Could you check a few things on this model? Use its own coordinates, in mm. A direction names the side the tool comes from. Give positions to 0.01 mm unless a question says otherwise; leave off trailing zeros. Order: outer loops, then holes, each group sorted by start corner. A loop starts at its lowest first (then second) coordinate and runs counter-clockwise, first axis right, second up.
Autodesk Fusion 360 part; units mm, degrees
sketch "Sketch1" plane through (0, 0, 0) normal (0, 0, 1) x (1, 0, 0)
  circle A0 centre (0, 0) radius 5
  circle A1 centre (0, 0) radius 3.575
  dimension "d1" = 10
  dimension "d2" = 7.15
extrude "Extrude1" add sketch "Sketch1" along normal blind 2
extrude "Extrude2" add sketch "Sketch1" along normal blind 4.9 contours A1
hole "Hole1" at (0, 0, 0) direction (0, 0, 1) diameter 5.5 depth 10 tip angle 118
Item 1: We'd pull the mould along X, two halves only. Please class faces 3 (the cylindrical face through (-1.08, 4.88, 0.99)), 4 (the flat face through (3.3, -2.2, 2)), 5 (the cylindrical face through (2.685, -0.596, 2.484)): +X half, -X half, draft (parallel to the pull), parting line (faces both ways), or undercut.
Findings:
face 3: parting line
face 4: draft
face 5: undercut
Item 2: Imagine slicing it at A-A on y = 0. List the corners of the cut face in (x, z) for me (3 decimals), then the cut area to 3 significant figures.
Findings:
outline: (-5, 0) - (-2.75, 0) - (-2.75, 4.9) - (-3.575, 4.9) - (-3.575, 2) - (-5, 2) - close; (2.75, 0) - (5, 0) - (5, 2) - (3.575, 2) - (3.575, 4.9) - (2.75, 4.9) - close
area: 13.8 mm2
Item 3: Imagine slicing it at D-D on y = -3.25. List the corners of the cut face in (x, z) for me.
Findings:
outline: (-3.8, 0) - (3.8, 0) - (3.8, 2) - (1.49, 2) - (1.49, 4.9) - (-1.49, 4.9) - (-1.49, 2) - (-3.8, 2) - close
Item 4: For faces 1 (the cylindrical face through (-0.465, -3.545, 3.43)), 2 (the flat face through (2.2, -2.2, 0)), which set-ups out of +Z, -Z, +X, -X, +Y, -Y let a thin tool reach every point of the face, with its end or its side?
Findings:
face 1: +Z
face 2: -Z, +X, -X, +Y, -Y
Item 5: Please list where these lines run through material, in increasing order: line 1 along Y through (x, z) = (0, 2.45) (3 decimals); line 2 along Y through (x, z) = (0, 1.85); line 3 along Z through (x, y) = (2.75, 2.75).
Findings:
line 1: y = -3.575 to -2.75, 2.75 to 3.575
line 2: y = -5 to -2.75, 2.75 to 5
line 3: z = 0 to 2
Item 6: Imagine slicing it at C-C on z = 2.65. List the corners of the cut face in (x, y) for me (3 decimals).
Findings:
outline: circle Ø7.15 at (0, 0); hole circle Ø5.5 at (0, 0)
